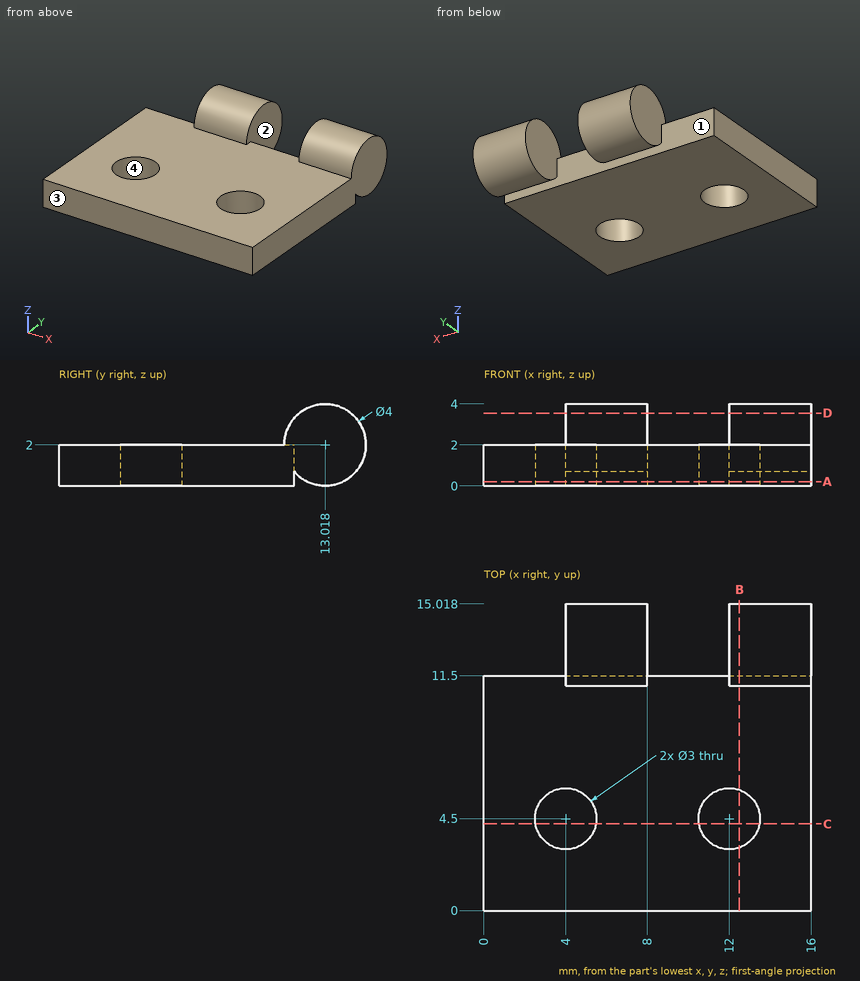
Input: dimensioned drawing with shaded views. Units: mm. Origin: part minimum x, y, z. Coordinates: 2 decimals unless noted, no trailing zeros. Loops run counter-clockwise (first coordinate to the right, second up) from the corner with the lowest first, then second, coordinate; pieces in that order, holes last.
Q1. Contact query for flat-ended pins moving along their axis: pin 1 (9 mm diameter, centred on x = 8, y = 5.5, fed in from +Z); pin 2 (1 mm diameter, centred on x = 7.5, z = 3.5, fed in from +Y); pin 3 (1.5 mm diameter, centred on x = 12, y = 11, fed in from +Z). Output: stop coordinate, or through.
Results are:
pin 1: stops at z = 2
pin 2: stops at y = 14.75
pin 3: stops at z = 3.55
Q2. Section A-A, the plane z = 0.2. Return the cut outline in (x, y).
Results are:
outline: (0, 0) - (16, 0) - (16, 11.5) - (0, 11.5) - close; (4, 12.15) - (8, 12.15) - (8, 13.89) - (4, 13.89) - close; (12, 12.15) - (16, 12.15) - (16, 13.89) - (12, 13.89) - close; hole circle Ø3 at (4, 4.5); hole circle Ø3 at (12, 4.5)
Q3. Section C-C, the plane y = 4.25. Return the cut outline in (x, z).
Results are:
outline: (0, 0) - (2.52, 0) - (2.52, 2) - (0, 2) - close; (5.48, 0) - (10.52, 0) - (10.52, 2) - (5.48, 2) - close; (13.48, 0) - (16, 0) - (16, 2) - (13.48, 2) - close
Q4. Line query: line 1 along X through (y, z) = (12, 3.1); line 2 along X through (y, z) = (3.25, 0.2); line 3 along Z through (x, y) = (14.5, 4). Output: solid intervals per line, ascending.
Results are:
line 1: x = 4 to 8, 12 to 16
line 2: x = 0 to 3.17, 4.83 to 11.17, 12.83 to 16
line 3: z = 0 to 2
Q5. Section D-D, the plane z = 3.55. Return the cut outline in (x, y).
Results are:
outline: (4, 11.75) - (8, 11.75) - (8, 14.28) - (4, 14.28) - close; (12, 11.75) - (16, 11.75) - (16, 14.28) - (12, 14.28) - close
Q6. Mould query, pull axis Y, two halves, no side actions, for the marked faces 1, 2, 3 and 4. Classes: +Y half, -Y half, draft (parallel to the pull), parting line (faces both ways), or undercut.
Results are:
face 1: undercut
face 2: draft
face 3: -Y half
face 4: undercut
Q7. Section B-B, the plane x = 12.5. Return the cut outline in (y, z), and give its area (3 significant figures).
Results are:
outline: (0, 0) - (3.09, 0) - (3.09, 2) - (0, 2) - close; (5.91, 0) - (11.5, 0) - (11.5, 0.7) arc R2 ccw (long way) to (11.02, 2) - (5.91, 2) - close
area: 29.5 mm2
